Geometry: see drawing. Coordinates: mm, zero at the bounding-box minimum. Round coordinates to 2 decimals unless told otherwise and drop trailing zeros. Order: outer loops, then holes, each group sorted by start corner. A loop starts at its lowest first (then second) coordinate and runs counter-clockwise, first axis right, second up. Notation, with made-up numbers: (51.25, 46) -> (56.25, 46) arc R18 ccw to (56.25, 72) -> close; hole circle Ø11 at (34, 24.5). An arc over 180 degrees is marked (long way). Put each result on its own line as item: value.
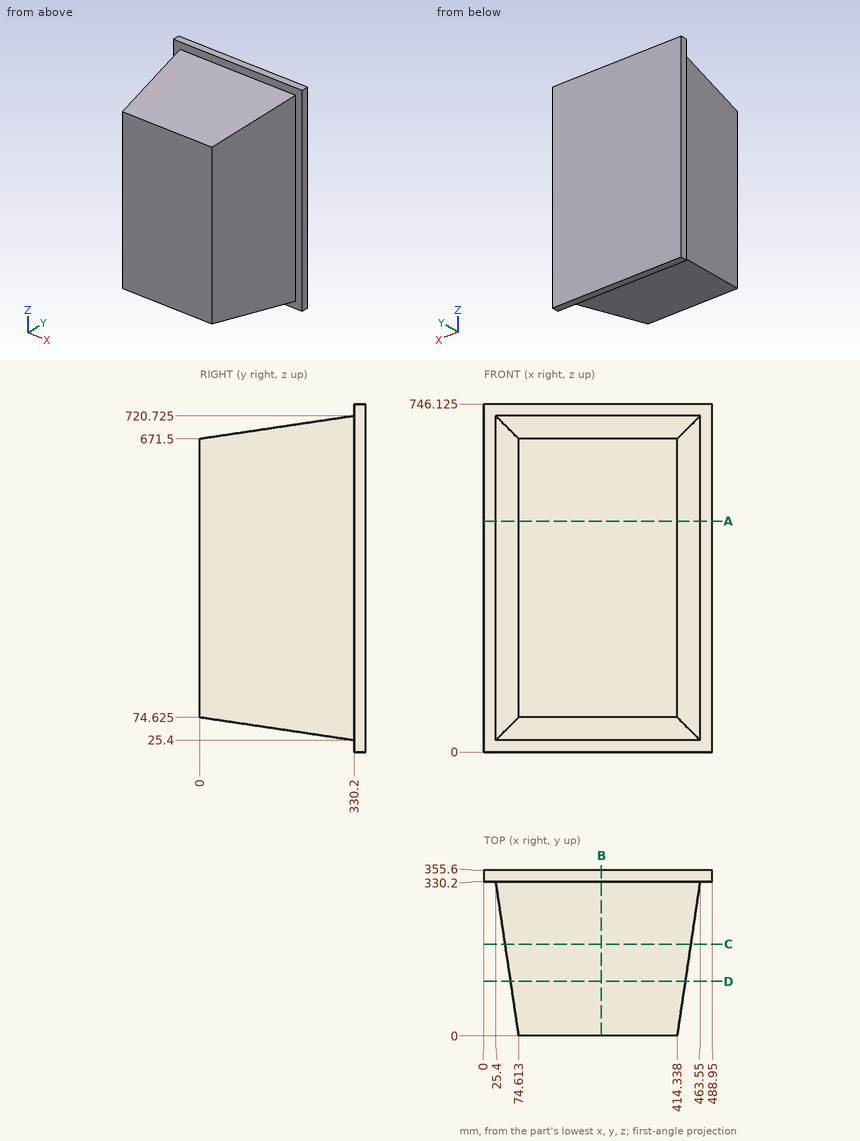
1. Cut plane C-C on y = 197. Return loops of the section in (x, z).
Ans:
outline: (45.25, 45.26) -> (443.7, 45.26) -> (443.7, 700.87) -> (45.25, 700.87) -> close
2. Cut plane B-B on x = 252. Return loops of the section in (y, z) (1 decimal).
Ans:
outline: (0, 74.6) -> (330.2, 25.4) -> (330.2, 0) -> (355.6, 0) -> (355.6, 746.1) -> (330.2, 746.1) -> (330.2, 720.7) -> (0, 671.5) -> close
3. Cut plane D-D on y = 117. Return loops of the section in (x, z) (1 decimal), and give its area (3 significant figures).
Ans:
outline: (57.2, 57.2) -> (431.8, 57.2) -> (431.8, 688.9) -> (57.2, 688.9) -> close
area: 237,000 mm²
4. Cut plane A-A on z = 495. Return loops of the section in (x, y).
Ans:
outline: (0, 330.2) -> (25.4, 330.2) -> (74.61, 0) -> (414.34, 0) -> (463.55, 330.2) -> (488.95, 330.2) -> (488.95, 355.6) -> (0, 355.6) -> close
5. Material intervals for probe 1 along Y at (x, z) = (20, 406.5); probe 2 along X at (y, z) = (216.5, 42.5) (1 decimal); probe 3 along Z at (x, y) = (287.5, 41.5), sorted ascending.
Ans:
probe 1: 330.2 to 355.6
probe 2: 42.3 to 446.6
probe 3: 68.44 to 677.69
6. Contact query for flat-ended pins moving along their axis: P1, Ø6, axis at y = 73.5, z = 146, coming from the +X side; P2, Ø2, axis at y = 118, z = 378.5, coming from the -X side; P3, Ø8, axis at x = 200.5, y = 176, coming from the -Z side. Output: stop coordinate, or through.
Ans:
P1: x = 425.74
P2: x = 56.88
P3: z = 47.79
